Autodesk Inventor part; units mm, degrees
ref_plane "YZ Plane" through (0, 0, 0) normal (1, 0, 0) x (0, 1, 0)
ref_plane "XZ Plane" through (0, 0, 0) normal (0, 1, 0) x (-1, 0, 0)
ref_plane "XY Plane" through (0, 0, 0) normal (0, 0, 1) x (1, 0, 0)
sketch "Эскиз1" plane through (0, 0, 0) normal (0, 1, 0) x (-1, 0, 0)
  line L0 (0, 0) -> (0, 15) construction
  line L1 (0, 15) -> (14.5, 15)
  line L2 (17, 12.5) -> (17, 1.75)
  line L3 (17, 1.75) -> (16.5, 1.75)
  line L4 (16.5, 1.75) -> (16.5, 12.5)
  line L5 (14.5, 14.5) -> (0, 14.5)
  line L6 (0, 14.5) -> (0, 15)
  arc A0 (16.5, 12.5) -> (14.5, 14.5) centre (14.5, 12.5) ccw
  arc A1 (17, 12.5) -> (14.5, 15) centre (14.5, 12.5) ccw
  line L7 (21.0213, 0) -> (-3.5036, 0)
  point P0 (17, 15)
  point P1 (16.5, 14.5)
  dimension "d0" = 15
  dimension "d1" = 17
  dimension "d2" = 13.25
  dimension "d3" = 0.5
  dimension "d4" = 12.75
  dimension "d5" = 2
  dimension "d6" = 2.5
revolve "Вращение1" add sketch "Эскиз1" angle 360 about axis through (-10, 0, 0) along (1, 0, 0)
properties part number "Кожух"
For this review, take the finished solid that the model builds, in its own axes (mm). Round coordinates to 2 decimals unless told otherwise and drop trailing zeros. Loops run counter-clockwise (first coordinate to the right, second up) from the corner with the lowest first, then second, coordinate; pieces in that order, holes last.
Q1. Mouldability with a two-part tool opening along Y and no side actions: class faces 1 (the face through (-16.746, 0.67, 1.617)), 2 (the face through (-17, 3, 0)), 3 (the face through (-7.352, 0.66, -14.985)) as +Y half, -Y half, draft (parallel to the pull), parting line (faces both ways), or undercut.
Result sheet:
face 1: undercut
face 2: draft
face 3: parting line
Q2. Add section C-C on x = -7.25. Write out the cut boundary in (y, z), plus the area to 3 significant figures.
Result sheet:
outline: circle Ø30 at (0, 0); hole circle Ø29 at (0, 0)
area: 46.3 mm2
Q3. Add section D-D on x = -15. Write out the cut boundary in (y, z), plus the area to 3 significant figures.
Result sheet:
outline: circle Ø29.9 at (0, 0); hole circle Ø28.87 at (0, 0)
area: 47.4 mm2
Q4. Add section A-A on y = 0. Write out the cut boundary in (x, z).
Result sheet:
outline: (-17, -12.5) arc R2.5 ccw to (-14.5, -15) - (0, -15) - (0, -14.5) - (-14.5, -14.5) arc R2 cw to (-16.5, -12.5) - (-16.5, -1.75) - (-17, -1.75) - close; (-17, 1.75) - (-16.5, 1.75) - (-16.5, 12.5) arc R2 cw to (-14.5, 14.5) - (0, 14.5) - (0, 15) - (-14.5, 15) arc R2.5 ccw to (-17, 12.5) - close
Q5. Insertion check: pin 1 Ø4 at (y, z) = (-4.5, -10.5) entering from +X; pin 2 Ø4 at (x, y) = (-6.5, 6.5) entering from -Z; pin 3 Ø3 at (x, y) = (-4.5, 6.5) entering from +Z. Each pin has a flat end and moves straight along its axis. Give the tip position at first contact, or say it passes through.
Result sheet:
pin 1: stops at x = -16.27
pin 2: stops at z = -14.31
pin 3: stops at z = 14.14
Q6. To check wall thickness, follow line 1 along Y through (x, z) = (-4, 0); line 2 along X through (y, z) = (-10.5, 2). State the ranges of each line that lie inside material, in increasing order.
Result sheet:
line 1: y = -15 to -14.5, 14.5 to 15
line 2: x = -17 to -16.5
